from build123d import *

# Parameters (mm, degrees)
EXTRUDE_1_DEPTH     = 61.4
SKETCH_2_W          = 17.963644186
SKETCH_2_H          = 5.547595999
SKETCH_2_W_2        = 22.810435624
SKETCH_2_H_2        = 6.55669033
CUT_EXTRUDE_1_DEPTH = 61.4
SKETCH_3_R          = 2
CUT_EXTRUDE_2_DEPTH = 2


with BuildPart() as part:
    # Эскиз1 → Вытянуть1 (new body)
    with BuildSketch(Plane.XY):
        Polygon((24.5, 0), (34, 0), (34, 23.7), (0, 23.7), (0, 0), (9.5, 0), (9.5, 10.7), (24.5, 10.7), align=None)
    extrude(amount=EXTRUDE_1_DEPTH)

    # Эскиз2 → Вырез-Вытянуть1 (cut)
    with BuildSketch(Plane(origin=(34, 0, 0), x_dir=(0, 0, -1), z_dir=(1, 0, 0))):
        with Locations((-59.381822093, 21.473798)):
            Rectangle(SKETCH_2_W, SKETCH_2_H)
        with Locations((0.405217812, 21.978345165)):
            Rectangle(SKETCH_2_W_2, SKETCH_2_H_2)
    extrude(amount=-CUT_EXTRUDE_1_DEPTH, mode=Mode.SUBTRACT)

    # Эскиз3 → Вырез-Вытянуть2 (cut)
    with BuildSketch(Plane(origin=(0, 23.7, 0), x_dir=(-1, 0, 0), z_dir=(0, 1, 0))):
        with Locations(Location((-4.0002, 17.6999, 0), (0, 0, 90))):
            Circle(SKETCH_3_R)
        with Locations(Location((-30.0002, 17.6999, 0), (0, 0, 90))):
            Circle(SKETCH_3_R)
        with Locations(Location((-4.0002, 43.6999, 0), (0, 0, 90))):
            Circle(SKETCH_3_R)
        with Locations(Location((-30.0002, 43.6999, 0), (0, 0, 90))):
            Circle(SKETCH_3_R)
    extrude(amount=-CUT_EXTRUDE_2_DEPTH, mode=Mode.SUBTRACT)


solid = part.part
Build history of the part. All positions in model axes, mm. A direction names the side the tool comes from. Give positions to 0.01 mm unless a question says otherwise; leave off trailing zeros. Order: outer loops, then holes, each group sorted by start corner. A loop starts at its lowest first (then second) coordinate and runs counter-clockwise, first axis right, second up. Notation, with made-up numbers: M 65,2.25 L 86,2.25 A20 ccw 86,8.25 Z; hole C -5,-10.75 d8. An arc over 180 degrees is marked long. Put each result on its own line as item: value.
Item 1: Cut at A-A on y = 5. Write the cut outline in (x, z), then the cut area to 3 significant figures.
Results are:
outline: M 0,0 L 9.5,0 L 9.5,61.4 L 0,61.4 Z; M 24.5,0 L 34,0 L 34,61.4 L 24.5,61.4 Z
area: 1,170 mm2
Item 2: Wall check: probe 1 along X at (y, z) = (2, 23); probe 2 along Y at (x, z) = (11.5, 8); probe 3 along Y at (x, z) = (21.5, 35). Give the ranges that are in metal, low to high.
Results are:
probe 1: 0 to 9.5, 24.5 to 34
probe 2: 10.7 to 18.7
probe 3: 10.7 to 23.7
Item 3: Cut at B-B on x = 8.5. Write the cut outline in (y, z), then the cut area to 3 significant figures.
Results are:
outline: M 0,0 L 18.7,0 L 18.7,11 L 23.7,11 L 23.7,50.4 L 18.7,50.4 L 18.7,61.4 L 0,61.4 Z
area: 1,350 mm2
Item 4: Which spindle directions (+Z, -Z, +X, -X, +Y, -Y) get a long thin tool onto all of the face, cutting with end or side? Do faces 1 (the face through (17, 10.7, 30)), 2 (the face through (17, 18.7, 6)), 3 (the face through (17, 21, 50.4)), 4 (the face through (4.09, 22.71, 41.7)). Say none if no direction does.
Results are:
face 1: +Z, -Z, -Y
face 2: -Z, +X, -X, +Y
face 3: +Z, +X, -X, +Y
face 4: +Y
Item 5: Drop flat-ended pins along their axis: pin 1 Ø1.2 at (x, z) = (5, 18) entering from +Y; pin 2 Ø8 at (x, z) = (16.5, 6.5) entering from -Y; pin 3 Ø5.5 at (x, z) = (19.5, 58) entering from +Y. Give the stop position or say it passes through.
Results are:
pin 1: y = 21.7
pin 2: y = 10.7
pin 3: y = 18.7
Item 6: Pull direction X, two halves, no side cores. Call faces 5 (the face through (34, 12, 30)), 6 (the face through (24.5, 5, 30)), 7 (the face through (17, 21, 11)), 8 (the face through (31.352, 22.714, 42.226)): +X half, -X half, draft (parallel to the pull), parting line (faces both ways), or undercut.
Results are:
face 5: +X half
face 6: undercut
face 7: draft
face 8: undercut
Item 7: Cut at D-D on y = 20.75. Write the cut outline in (x, z), then the cut area to 3 significant figures.
Results are:
outline: M 0,11 L 34,11 L 34,50.4 L 0,50.4 Z
area: 1,340 mm2
Item 8: Cut at C-C on z = 47. Write the cut outline in (x, y), then the cut area to 3 significant figures.
Results are:
outline: M 0,0 L 9.5,0 L 9.5,10.7 L 24.5,10.7 L 24.5,0 L 34,0 L 34,23.7 L 0,23.7 Z
area: 645 mm2
